```python
from build123d import *

# Parameters (mm, degrees)
CHAMFER1_SIZE      = 0.8
CHAMFER2_SIZE      = 0.5
CUT_EXTRUDE1_DEPTH = 2.5
CHAMFER3_SIZE      = 0.4


with BuildPart() as part:
    # Sketch1 → Revolve1 (revolve)
    with BuildSketch(Plane.XY):
        Polygon((0, 0), (0, 4.25), (5, 4.25), (5, 2.488), (28, 2.488), (28, 0), align=None)
    revolve(axis=Axis((-88.705490849, 0, 0), (1, 0, 0)))

    # Chamfer1
    chamfer1_edges = [part.edges().sort_by_distance(p)[0] for p in [
        (28, -2.488, 0),
    ]]
    chamfer(chamfer1_edges, length=CHAMFER1_SIZE)

    # Chamfer2
    chamfer2_edges = [part.edges().sort_by_distance(p)[0] for p in [
        (0, -4.25, 0),
    ]]
    chamfer(chamfer2_edges, length=CHAMFER2_SIZE)

    # Sketch3 → Cut-Extrude1 (cut)
    with BuildSketch(Plane(origin=(0, 0, 0), x_dir=(0, 0, -1), z_dir=(1, 0, 0))):
        Polygon((-2.309401077, 0), (-1.154700538, -2), (1.154700538, -2), (2.309401077, 0), (1.154700538, 2), (-1.154700538, 2), align=None)
    extrude(amount=CUT_EXTRUDE1_DEPTH, mode=Mode.SUBTRACT)

    # Chamfer3
    chamfer3_edges = [part.edges().sort_by_distance(p)[0] for p in [
        (0, 1, 1.732050808),
        (0, -1, 1.732050808),
        (0, -2, 0),
        (0, -1, -1.732050808),
        (0, 1, -1.732050808),
        (0, 2, 0),
    ]]
    chamfer(chamfer3_edges, length=CHAMFER3_SIZE)


solid = part.part
```
Geometry check sheet. Reference: the model listing, model coordinates, mm. A direction names the side the tool comes from. Round coordinates to 2 decimals unless told otherwise and drop trailing zeros. Loops run counter-clockwise (first coordinate to the right, second up) from the corner with the lowest first, then second, coordinate; pieces in that order, holes last. Notation, with made-up numbers: M 44,27 L 95,27 A35 cw 95,65 Z; hole C 7,6 d10. An arc over 180 degrees is marked long. Return JSON: item names as keys, results as strings. Group by question number.
(1) Mould release check, pull along Z, two halves, no side actions. Record for faces 1 (the face through (1.44, 0.99, -1.74)), 2 (the face through (0.203, -1.082, 1.913)), 3 (the face through (2.782, 2.285, 3.584)), 4 (the face through (5, 2, -2)): pulls with the +Z half, pulls with the -Z half, needs draft (parallel to the pull), parting line crosses it, or undercut.
(2) Set-up check for faces 5 (the face through (0, 0.89, -2.45)), 6 (the face through (16.255, 2.373, 0.747)), 7 (the face through (0.203, 1.115, 1.893)): record each of +Z, -Z, +X, -X, +Y, -Y from which the full face is reachable in a straight line by a thin tool's end or side.
(3) Section check C-C, the plane x = 24. Enter the section's corners in (y, z), and give its area (3 significant figures).
(4) Scan lines: line 1 along X through (y, z) = (3.5, -0.75); line 2 along X through (y, z) = (-1, 1); line 3 along Y through (x, z) = (25.25, 0.25). Record each from-to range of solid material in increasing order. Write a range as [from, to].
(5) Go/stop test with flat-tipped pins: pin 1 (2 mm diameter, centred on x = 7.5, y = 2.5, fed in from -Z) (3 decimals); pin 2 (3 mm diameter, centred on y = 0.5, z = 0.5, fed in from -X); pin 3 (3 mm diameter, centred on x = 8, y = -3.5, fed in from -Z). Record where each tip stops, or that it passes through.
(6) Section check B-B, the plane x = 4.25. Enter the section's corners in (y, z), and give its area (3 significant figures).
(7) Section check A-A, the plane z = 0. Enter the section's corners in (x, y), and give its area (3 significant figures).
Data:
{
 "1": {"face 1": "undercut", "face 2": "undercut", "face 3": "parting line crosses it", "face 4": "needs draft"},
 "2": {"face 5": "+Z, -Z, -X, +Y, -Y", "face 6": "+X", "face 7": "-X"},
 "3": {"outline": "C 0,0 d4.98", "area": "19.4 mm²"},
 "4": {"line 1": "[0, 5]", "line 2": "[2.5, 28]", "line 3": "[-2.48, 2.48]"},
 "5": {"pin 1": "z = -1.985", "pin 2": "x = 0.22", "pin 3": "z = -1.48"},
 "6": {"outline": "C 0,0 d8.5", "area": "56.7 mm²"},
 "7": {"outline": "M 0,-3.75 L 0.5,-4.25 L 5,-4.25 L 5,-2.49 L 27.2,-2.49 L 28,-1.69 L 28,1.69 L 27.2,2.49 L 5,2.49 L 5,4.25 L 0.5,4.25 L 0,3.75 L 0,2.4 L 0.4,2 L 2.5,2 L 2.5,-2 L 0.4,-2 L 0,-2.4 Z", "area": "146 mm²"}
}
